The listing builds one solid part. Answer for the finished solid, in the listing's coordinates (mm). A direction names the side the tool comes from. Round coordinates to 2 decimals unless told otherwise and drop trailing zeros. Loops run counter-clockwise (first coordinate to the right, second up) from the corner with the lowest first, then second, coordinate; pieces in that order, holes last. Notation, with made-up numbers: M 28,-28 L 81,-28 A14 ccw 81,-13 Z; hole C 21.5,15 d5. An arc over 180 degrees is marked long. Answer as a JSON object with one key per item and string values.
```python
from build123d import *

# Parameters (mm, degrees)
EXTRUDE_1_DEPTH     = 8
SKETCH_2_W          = 7
SKETCH_2_H          = 60
EXTRUDE_2_DEPTH     = 22
MM_1_D              = 9
CUT_EXTRUDE_1_DEPTH = 22
HOLE_WIZARD_M5_1_D  = 4.2


with BuildPart() as part:
    # 草图1 → 凸台-拉伸1 (new body)
    with BuildSketch(Plane(origin=(0, 0, 0), x_dir=(1, 0, 0), z_dir=(0, 1, 0))):
        with BuildLine():
            Line((-14.75, 30), (40.25, 30))
            Line((40.25, 30), (40.25, -30))
            Line((40.25, -30), (-14.75, -30))
            ThreePointArc((-14.75, -30), (-44.75, 0), (-14.75, 30))
        make_face()
    extrude(amount=EXTRUDE_1_DEPTH)

    # 草图2 → 凸台-拉伸2 (add)
    with BuildSketch(Plane(origin=(0, 8, 0), x_dir=(1, 0, 0), z_dir=(0, 1, 0))):
        with Locations((36.75, 0)):
            Rectangle(SKETCH_2_W, SKETCH_2_H)
    extrude(amount=EXTRUDE_2_DEPTH)

    # 大小mm 暗销孔1 (through all)
    with Locations(Plane(origin=(40.25, 15, 15), x_dir=(0, 0, 1), z_dir=(1, 0, 0))):
        with Locations((0, 0), (-30, 0)):
            Hole(MM_1_D / 2)

    # 草图5 → 切除-拉伸1 (cut)
    with BuildSketch(Plane.XZ):
        with BuildLine():
            Line((-27.75, 9), (10.25, 9))
            ThreePointArc((10.25, 9), (19.25, 0), (10.25, -9))
            Line((10.25, -9), (-27.75, -9))
            ThreePointArc((-27.75, -9), (-36.75, 0), (-27.75, 9))
        make_face()
    extrude(amount=-CUT_EXTRUDE_1_DEPTH, mode=Mode.SUBTRACT)

    # M5 螺纹孔1 (through all)
    with Locations(Plane(origin=(-31.75, 0, 15), x_dir=(0, 0, -1), z_dir=(0, -1, 0))):
        with Locations((0, 0), (0, 50), (30, 50), (30, 0)):
            Hole(HOLE_WIZARD_M5_1_D / 2)


solid = part.part
```
Item 1: Straight lines are drawn through the part: line 1 (X direction, y = 1.5, z = 0); line 2 (Y direction, x = 38.75, z = 15); line 3 (X direction, y = 12.75, z = -0.5). For each, find the intervals that lie inside material, in ascending order.
Values follow:
{"line 1": "-44.75 to -36.75, 19.25 to 40.25", "line 2": "0 to 10.5, 19.5 to 30", "line 3": "33.25 to 40.25"}
Item 2: The part is cut by section C-C (z = 0). Give the vertices of the cut face in (x, y).
Values follow:
{"outline": "M -44.75,0 L -36.75,0 L -36.75,8 L -44.75,8 Z; M 19.25,0 L 40.25,0 L 40.25,30 L 33.25,30 L 33.25,8 L 19.25,8 Z"}
Item 3: The part is cut by section B-B (y = 15). Give the vertices of the cut face in (x, z).
Values follow:
{"outline": "M 33.25,-30 L 40.25,-30 L 40.25,-19.5 L 33.25,-19.5 Z; M 33.25,-10.5 L 40.25,-10.5 L 40.25,10.5 L 33.25,10.5 Z; M 33.25,19.5 L 40.25,19.5 L 40.25,30 L 33.25,30 Z"}
Item 4: The part is cut by section D-D (y = 6). Give the vertices of the cut face in (x, z), then the cut area to 3 significant figures.
Values follow:
{"outline": "M -14.75,-30 L 40.25,-30 L 40.25,30 L -14.75,30 A30 ccw Z; hole C -31.75,-15 d4.2; hole C -31.75,15 d4.2; hole M -27.75,-9 L 10.25,-9 A9 ccw 10.25,9 L -27.75,9 A9 ccw Z; hole C 18.25,-15 d4.2; hole C 18.25,15 d4.2", "area": "3,720 mm^2"}
Item 5: The part is cut by section A-A (x = 1.5). Give the vertices of the cut face in (y, z), then the cut area to 3 significant figures.
Values follow:
{"outline": "M 0,-30 L 8,-30 L 8,-9 L 0,-9 Z; M 0,9 L 8,9 L 8,30 L 0,30 Z", "area": "336 mm^2"}
Item 6: Flat-ended cylindrical pins translate along their axes: P1, Ø6.5, axis at x = 18.25, z = 15, coming from the +Y side; P2, Ø6.5, axis at y = 20.5, z = 0.5, coming from the -X side. Find the tip coordinate at first contact, or state that the pin passes through.
Values follow:
{"P1": "y = 8", "P2": "x = 33.25"}
Item 7: Which of the six approach directions +Z, -Z, +X, -X, +Y, -Y give full straight-line access (tool end or side, diameter ignored) to faces 1 (the face through (17, 7, -30)), 2 (the face through (-9, 4, 9)), 3 (the face through (3, 8, 13))?
Values follow:
{"face 1": "-Z, +X, -X, +Y, -Y", "face 2": "+Y, -Y", "face 3": "+Z, -Z, -X, +Y"}
Item 8: Determine the mould class of faces 4 (the face through (36.7, 10.54, -14.41)), 5 (the face through (17, 7, 30)), 6 (the face through (33.25, 19, 0)), 7 (the face through (20.02, 4.06, -13.87)) for opening direction Z: released by +Z, released by -Z, zero draft, split by the parting line, or undercut.
Values follow:
{"face 4": "undercut", "face 5": "released by +Z", "face 6": "zero draft", "face 7": "undercut"}
